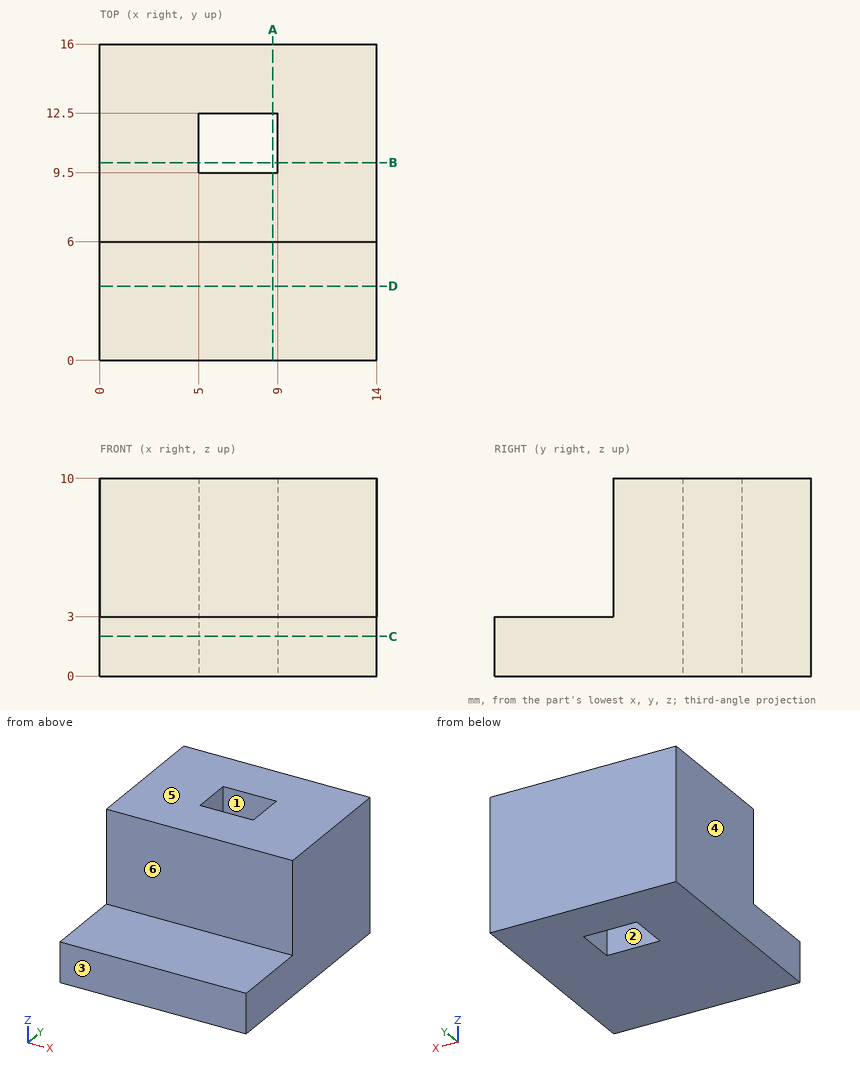
The figure shows three views and two pictorial views of one solid part (mm, origin at its lowest corner). Answer the questions. A direction names the side the tool comes from. Give positions to 0.01 mm unless a question says otherwise; leave off trailing zeros. Write each loop counter-clockwise with the first axis right and the second up, starting at its lowest first coordinate (ties: lowest second). Pieces come first, ordered by that corner, then holes. Notation, with made-up numbers: M 37.25,30 L 63.25,30 A25 ccw 63.25,50 Z; hole C 62.25,-7 d10. An arc over 180 degrees is marked long. One line per item, written item: value. Start each with the question number.
(1) Find section B-B (y = 10). Determine the outline of the cut face in (x, z), plus the area to 3 significant figures.
(2) Determine the mould class of the marked faces 1, 2, 3 and 4 for opening direction Y: pulls with the +Y half, pulls with the -Y half, needs draft (parallel to the pull), parting line crosses it, or undercut.
(3) A flat-ended cylindrical pin translates along its axis: pin 1 Ø3 at (x, z) = (10, 8.5) entering from -Y. Find the tip coordinate at first contact, or state that the pin passes through.
(4) A tool of negligible diameter and unlimited length cuts with its end or side. For the marked faces 5 and 6, from which of +Z, -Z, +X, -X, +Y, -Y can it reach the whole face along a straight path? Write none if from no direction.
(5) Find section C-C (z = 2). Determine the outline of the cut face in (x, y).
(6) Find the intervals of material crossed by line 1 (Y direction, x = 7, z = 9); line 2 (Y direction, x = 5.75, z = 2.25); line 3 (X direction, y = 11.5, z = 6.5), in increasing order.
(7) Find section A-A (x = 8.75). Determine the outline of the cut face in (y, z), plus the area to 3 significant figures.
(8) Find section D-D (y = 3.75). Determine the outline of the cut face in (x, z).
Results below:
1. outline: M 0,0 L 5,0 L 5,10 L 0,10 Z; M 9,0 L 14,0 L 14,10 L 9,10 Z
1. area: 100 mm^2
2. face 1: undercut
2. face 2: undercut
2. face 3: pulls with the -Y half
2. face 4: needs draft
3. pin 1: stops at y = 6
4. face 5: +Z, +X, -X, +Y, -Y
4. face 6: +Z, +X, -X, -Y
5. outline: M 0,0 L 14,0 L 14,16 L 0,16 Z; hole M 5,9.5 L 9,9.5 L 9,12.5 L 5,12.5 Z
6. line 1: y = 6 to 9.5, 12.5 to 16
6. line 2: y = 0 to 9.5, 12.5 to 16
6. line 3: x = 0 to 5, 9 to 14
7. outline: M 0,0 L 9.5,0 L 9.5,10 L 6,10 L 6,3 L 0,3 Z; M 12.5,0 L 16,0 L 16,10 L 12.5,10 Z
7. area: 88.0 mm^2
8. outline: M 0,0 L 14,0 L 14,3 L 0,3 Z
